Geometry: final body of the model. Coordinates: model frame, mm. Face numbers are marked on the shaded views. A direction names the side the tool comes from. Round coordinates to 2 decimals unless told otherwise and drop trailing zeros. Loops run counter-clockwise (first coordinate to the right, second up) from the corner with the lowest first, then second, coordinate; pieces in that order, holes last. Notation, with made-up numbers: M 33.5,12 L 41.5,12 A31 ccw 41.5,49 Z; hole C 36.5,45 d8. An arc over 180 degrees is marked long. Return JSON: item names as keys, results as strings.
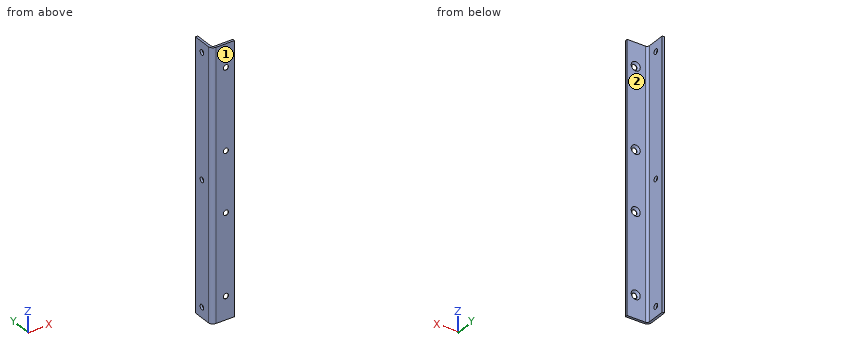
from build123d import *

# Parameters (mm, degrees)
EXTRUDE_1_DEPTH     = 232
SKETCH_2_R          = 2.25
CUT_EXTRUDE_1_DEPTH = 10
SKETCH_3_R          = 2.25
CUT_EXTRUDE_2_DEPTH = 10
CHAMFER_1_SIZE      = 1.7
FILLET_1_R          = 4


with BuildPart() as part:
    # Эскиз1 → Вытянуть1 (new body)
    with BuildSketch(Plane.XY):
        with BuildLine():
            Line((0, 0), (20, 0))
            Line((20, 0), (20, 2))
            Line((20, 2), (4, 2))
            ThreePointArc((4, 2), (2.585786438, 2.585786438), (2, 4))
            Line((2, 4), (2, 20))
            Line((2, 20), (0, 20))
            Line((0, 20), (0, 0))
        make_face()
    extrude(amount=EXTRUDE_1_DEPTH)

    # Эскиз2 → Вырез-Вытянуть1 (cut)
    with BuildSketch(Plane(origin=(2, 0, 0), x_dir=(0, 0, -1), z_dir=(1, 0, 0))):
        with Locations((-223, 12)):
            Circle(SKETCH_2_R)
        with Locations((-9, 12)):
            Circle(SKETCH_2_R)
        with Locations((-116, 12)):
            Circle(SKETCH_2_R)
    extrude(amount=-CUT_EXTRUDE_1_DEPTH, mode=Mode.SUBTRACT)

    # Эскиз3 → Вырез-Вытянуть2 (cut)
    with BuildSketch(Plane(origin=(0, 2, 0), x_dir=(1, 0, 0), z_dir=(0, 1, 0))):
        with Locations(Location((12.5, -212, 0), (0, 0, 270))):
            Circle(SKETCH_3_R)
        with Locations(Location((12.5, -142, 0), (0, 0, 270))):
            Circle(SKETCH_3_R)
        with Locations(Location((12.5, -20, 0), (0, 0, 270))):
            Circle(SKETCH_3_R)
        with Locations(Location((12.5, -90, 0), (0, 0, 270))):
            Circle(SKETCH_3_R)
    extrude(amount=-CUT_EXTRUDE_2_DEPTH, mode=Mode.SUBTRACT)

    # Фаска1
    chamfer_1_edges = [part.edges().sort_by_distance(p)[0] for p in [
        (12.5, 2, 209.75),
        (12.5, 2, 139.75),
        (12.5, 2, 17.75),
        (12.5, 2, 87.75),
    ]]
    chamfer(chamfer_1_edges, length=CHAMFER_1_SIZE)

    # Скругление1
    fillet_1_edges = [part.edges().sort_by_distance(p)[0] for p in [
        (0, 0, 116),
    ]]
    fillet(fillet_1_edges, radius=FILLET_1_R)


solid = part.part
Q1. Pin query (flat end, axial travel): pin 1 (4 mm diameter, centred on x = 18, y = 4.5, fed in from -Z); pin 2 (1 mm diameter, centred on y = 12, z = 71, fed in from +X); pin 3 (5 mm diameter, centred on x = 15, z = 66, fed in from +Y). Return the tip coordinate at first contact, or that it passes through.
Determined:
{"pin 1": "passes through", "pin 2": "stops at x = 2", "pin 3": "stops at y = 2"}
Q2. Section query A-A (y = 12). Output: boundary loops of the cut face in (x, z), plus the area to 3 significant figures.
Determined:
{"outline": "M 0,0 L 2,0 L 2,6.75 L 0,6.75 Z; M 0,11.25 L 2,11.25 L 2,113.75 L 0,113.75 Z; M 0,118.25 L 2,118.25 L 2,220.75 L 0,220.75 Z; M 0,225.25 L 2,225.25 L 2,232 L 0,232 Z", "area": "437 mm^2"}
Q3. Section query B-B (z = 9). Output: boundary loops of the cut face in (x, y), plus the area to 3 significant figures.
Determined:
{"outline": "M 0,4 A4 ccw 4,0 L 20,0 L 20,2 L 4,2 A2 cw 2,4 L 2,9.75 L 0,9.75 Z; M 0,14.25 L 2,14.25 L 2,20 L 0,20 Z", "area": "64.4 mm^2"}
Q4. Section query C-C (z = 105.5). Output: boundary loops of the cut face in (x, y), plus the area to 3 significant figures.
Determined:
{"outline": "M 0,4 A4 ccw 4,0 L 20,0 L 20,2 L 4,2 A2 cw 2,4 L 2,20 L 0,20 Z", "area": "73.4 mm^2"}
Q5. Material intervals for L1, parallel to Z at x = 11, y = 1; L2, parallel to Y at x = 0.55, z = 9; L3, parallel to Y at x = 10.5, z = 124.5, sorted ascending.
Determined:
{"L1": "z = 0 to 17.46, 22.54 to 87.46, 92.54 to 139.46, 144.54 to 209.46, 214.54 to 232", "L2": "y = 1.98 to 9.75, 14.25 to 20", "L3": "y = 0 to 2"}
Q6. Reachability of the marked faces 1 and 2 from +Z, -Z, +X, -X, +Y, -Y: full face, straight path, thin tool, end or side. Return the list, or none.
Determined:
{"face 1": "+Z, -Z, +X, -X, -Y", "face 2": "+Z, -Z, +X, +Y"}
